from build123d import *

# Parameters (mm, degrees)
SKETCH_R      = 5
SKETCH_R_2    = 6.5
EXTRUDE_DEPTH = 8


with BuildPart() as part:
    # Sketch → Extrude (new body)
    with BuildSketch(Plane.XY):
        Polygon((92.138212, 71.477997), (99.138212, 59.353641), (104.147683, 60.457133), (108.020931, 58.166292), (109.466872, 53.244732), (104.121576, 44.207154), (96.375081, 48.788836), (90.266171, 38.460176), (98.012666, 33.878494), (92.66737, 24.840916), (87.657898, 23.737425), (83.784651, 26.028266), (82.33871, 30.949826), (68.33871, 30.949826), (66.794519, 26.058201), (62.873968, 23.849291), (57.887594, 25.052863), (52.731628, 34.204082), (60.572729, 38.621903), (54.682302, 49.076704), (46.841201, 44.658884), (41.688919, 53.803566), (43.23311, 58.695191), (47.15366, 60.904101), (52.140035, 59.700529), (59.140035, 71.824885), (55.679647, 75.611469), (55.72695, 80.11122), (59.266176, 83.824222), (69.765596, 83.713849), (69.67099, 74.714346), (81.670327, 74.588205), (81.764933, 83.587708), (92.264353, 83.477334), (95.72474, 79.69075), (95.677437, 75.190999), align=None)
        with Locations((76.588238, 60.640856)):
            Circle(SKETCH_R, mode=Mode.SUBTRACT)
        with Locations((64.201959, 52.770623)):
            Circle(SKETCH_R_2, mode=Mode.SUBTRACT)
        with Locations((88.200633, 52.51834)):
            Circle(SKETCH_R_2, mode=Mode.SUBTRACT)
    extrude(amount=EXTRUDE_DEPTH)


solid = part.part
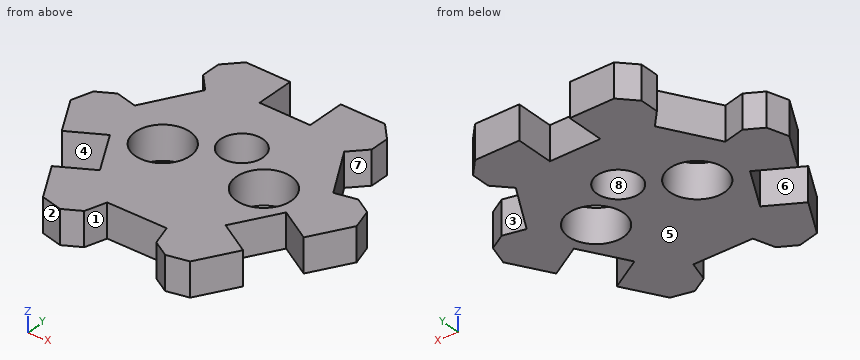
The model under review builds one solid part; all positions refer to its coordinate system, in mm. Face numbers are marked on the shaded views. A direction names the side the tool comes from. Round coordinates to 2 decimals unless told otherwise and drop trailing zeros. Write each loop counter-clockwise with the first axis right and the second up, starting at its lowest first coordinate (ties: lowest second). Pieces come first, ordered by that corner, then holes. Notation, with made-up numbers: M 71,-31.75 L 110,-31.75 A10 cw 110,-16.75 Z; hole C 82.5,-27 d5. An arc over 180 degrees is marked long. Use a Markdown table: item, result. Add a question column.
Q1. To check wall thickness, follow line 1 (X direction, y = 50, z = 7); line 2 (Y direction, x = 95.5, z = 0.5); line 3 (X direction, y = 58, z = 2). State the ranges of each line that lie inside material, in increasing order.
Q2. Machinability: for the marked faces 1, 2, 3, 4 and 5, which of the approach directions +Z, -Z, +X, -X, +Y, -Y give a long, thin tool a straight path to every point of the face, cutting with its end or side? Answer none if there is none.
Q3. We need section C-C, the plane x = 64. State the section outline as (y, z) points.
Q4. We need section D-D, the plane z = 7. Count the separate pieces of the cut face and the enclosed holes in it, plus the area to 3 significant figures.
Q5. The part is to be moulded in two halves that separate along X. For the marked faces 6, 7 and 8, say which applies: pulls with the +X half, pulls with the -X half, needs draft (parallel to the pull), parting line crosses it, or undercut.
Q6. Insertion check: pin 1 (3 mm diameter, centred on y = 31, z = 2.5, fed in from -X); pin 2 (1.5 mm diameter, centred on y = 52, z = 3.5, fed in from -X); pin 3 (2.5 mm diameter, centred on x = 77.5, z = 4, fed in from -Y). Each pin has a flat end and moves straight along its axis. Give the tip position at first contact, or say it passes through.
Q7. We need section A-A, the plane x = 80. State the section outline as (y, z) points, plus the area to 3 significant figures.
Q8. We need section B-B, the plane y = 57. State the section outline as (x, z) points.
Findings below:
| question | item | result |
|---|---|---|
| 1 | line 1 | x = 43.83 to 58.32, 70.08 to 82.21, 94.19 to 107.55 |
| 1 | line 2 | y = 29.63 to 35.36, 47.31 to 65.66, 75 to 79.94 |
| 1 | line 3 | x = 43.01 to 60.34, 68.06 to 72.34, 80.83 to 84.71, 91.69 to 108.07 |
| 2 | face 1 | +Z, -Z, -Y |
| 2 | face 2 | +Z, -Z, -X, -Y |
| 2 | face 3 | +Z, -Z, +Y |
| 2 | face 4 | +Z, -Z |
| 2 | face 5 | -Z, +X, -X, +Y, -Y |
| 3 | outline | M 24.48,0 L 46.27,0 L 46.27,8 L 24.48,8 Z; M 59.27,0 L 83.77,0 L 83.77,8 L 59.27,8 Z |
| 4 | separate pieces | 1 |
| 4 | enclosed holes | 3 |
| 4 | area | 2,050 mm² |
| 5 | face 6 | pulls with the -X half |
| 5 | face 7 | pulls with the +X half |
| 5 | face 8 | undercut |
| 6 | pin 1 | stops at x = 53.69 |
| 6 | pin 2 | stops at x = 42.28 |
| 6 | pin 3 | stops at y = 30.95 |
| 7 | outline | M 30.95,0 L 56.99,0 L 56.99,8 L 30.95,8 Z; M 64.3,0 L 74.61,0 L 74.61,8 L 64.3,8 Z |
| 7 | area | 291 mm² |
| 8 | outline | M 42.7,0 L 59.27,0 L 59.27,8 L 42.7,8 Z; M 69.14,0 L 73.16,0 L 73.16,8 L 69.14,8 Z; M 80.02,0 L 83.49,0 L 83.49,8 L 80.02,8 Z; M 92.91,0 L 108.36,0 L 108.36,8 L 92.91,8 Z |
